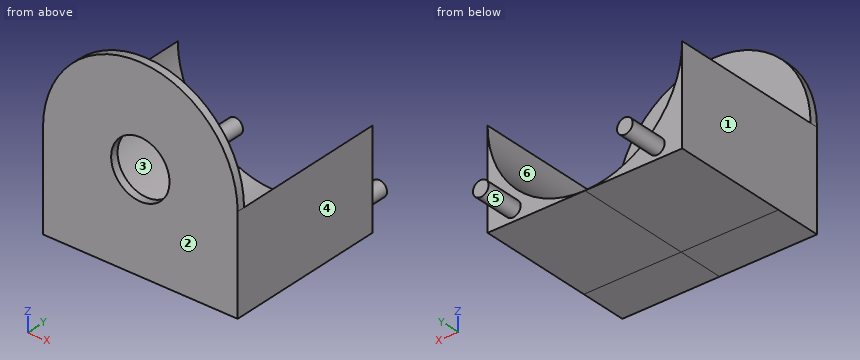
Autodesk Inventor part; units mm, degrees
ref_plane "YZ Plane" through (0, 0, 0) normal (1, 0, 0) x (0, 1, 0)
ref_plane "XZ Plane" through (0, 0, 0) normal (0, 1, 0) x (-1, 0, 0)
ref_plane "XY Plane" through (0, 0, 0) normal (0, 0, 1) x (1, 0, 0)
sketch "Sketch1" plane through (0, 0, 0) normal (0, 1, 0) x (-1, 0, 0)
  circle A0 centre (0, 0) radius 7.5
  circle A1 centre (0, 0) radius 25
  dimension "d0" = 15
  dimension "d1" = 50
extrude "Extrusion1" add sketch "Sketch1" along normal blind 2
sketch "Sketch2" plane through (0, 2, 0) normal (0, 1, 0) x (1, 0, 0)
  circle A0 centre (0, 0) radius 25
  line L0 (25, 0) -> (-25, 0)
  line L1 (-25, 0) -> (-25, 25)
  line L2 (-25, 25) -> (25, 25)
  line L3 (25, 25) -> (25, 0)
  point P0 (0, 25)
extrude "Extrusion2" add sketch "Sketch2" along normal blind 10 and the other way blind 2 contours L1 L2 A0 | A0 L2 L3
sketch "Sketch3" plane through (0, 12, 0) normal (0, 1, 0) x (1, 0, 0)
  circle A0 centre (21.5, 18.5) radius 2
  circle A1 centre (-21.5, 18.5) radius 2
  point P0 (0, 0)
  dimension "d8" = 4
  dimension "d9" = 4
extrude "Extrusion3" add sketch "Sketch3" along normal blind 40
sketch "Sketch4" plane through (0, 0, 0) normal (0, -1, 0) x (1, 0, 0)
  line L0 (25, -25) -> (0, -25)
  arc A0 (25, 0) -> (-25, 0) centre (0, 0) ccw
  line L1 (25, -25) -> (-25, -25)
  line L2 (-25, -25) -> (-25, 0)
  line L3 (-25, 0) -> (25, 0)
  line L4 (25, 0) -> (25, -25)
  arc A1 (0, -25) -> (25, 0) centre (0, 0) ccw
  arc A2 (-25, 0) -> (25, 0) centre (0, 0) ccw
extrude "Extrusion4" add sketch "Sketch4" against normal blind 42 contours L0 A1 L4 | L1 L2 A2
sketch "Sketch5" plane through (21.5, 52, -18.5) normal (0, 1, 0) x (1, 0, 0)
  circle A0 centre (0, 0) radius 2
  circle A1 centre (0, 0) radius 2
  circle A2 centre (-43, 0) radius 2
  circle A3 centre (-43, 0) radius 2
  point P0 (-21.5, -18.5)
extrude "Extrusion5" cut sketch "Sketch5" against normal blind 10
sketch "Sketch6" plane through (0, 42, 0) normal (0, 1, 0) x (1, 0, 0)
  circle A0 centre (18.5, 22) radius 2
  circle A1 centre (-18.5, 22) radius 2
  point P0 (0, 0)
  dimension "d16" = 4
  dimension "d17" = 4
extrude "Extrusion6" add sketch "Sketch6" along normal blind 10
properties part number "trail 3.1" material "Iron, Gray"
Geometry: final body of the model. Coordinates: model frame, mm. Face numbers are marked on the shaded views. A direction names the side the tool comes from. Give positions to 0.01 mm unless a question says otherwise; leave off trailing zeros. Write each loop counter-clockwise with the first axis right and the second up, starting at its lowest first coordinate (ties: lowest second). Pieces come first, ordered by that corner, then holes. Notation, with made-up numbers: (-2, -20.5) -> (11, -20.5) arc R28 cw to (11, -2.5) -> close; hole circle Ø11 at (61.5, 55.25). An arc over 180 degrees is marked (long way). Answer in a Markdown table with one row per item.
(1) Section query C-C on x = -18.5. Return loops of the section in (y, z), then the cut area to 3 significant figures.
Answers below:
| item | result |
|---|---|
| outline | (0, -25) -> (42, -25) -> (42, -24) -> (52, -24) -> (52, -20) -> (42, -20) -> (42, -16.82) -> (2, -16.82) -> (2, 16.82) -> (0, 16.82) -> close |
| area | 451 mm^2 |
(2) Section query D-D on z = -14. Return loops of the section in (x, y), then the cut area to 3 significant figures.
Answers below:
| item | result |
|---|---|
| outline | (-25, 0) -> (25, 0) -> (25, 42) -> (20.71, 42) -> (20.71, 2) -> (-20.71, 2) -> (-20.71, 42) -> (-25, 42) -> close |
| area | 443 mm^2 |
(3) Ray query, line 1 along Z through (x, y) = (0, 1.45); line 2 along Y through (x, z) = (15, 14.5); line 3 along X through (y, z) = (22, -21.5). Return the intervals inside material, ascending. Write a range as [from, to].
Answers below:
| item | result |
|---|---|
| line 1 | [-25, -7.5], [7.5, 25] |
| line 2 | [0, 2] |
| line 3 | [-25, -12.76], [12.76, 25] |
(4) Section query A-A on z = 3. Return loops of the section in (x, y), then the cut area to 3 significant figures.
Answers below:
| item | result |
|---|---|
| outline | (-24.82, 0) -> (-6.87, 0) -> (-6.87, 2) -> (-24.82, 2) -> close; (6.87, 0) -> (24.82, 0) -> (24.82, 2) -> (6.87, 2) -> close |
| area | 71.8 mm^2 |
(5) Pin query (flat end, axial travel): pin 1 (5 mm diameter, centred on x = -11, z = -11.5, fed in from +Y); pin 2 (10 mm diameter, centred on x = 1, y = 25.5, fed in from +Z); pin 3 (12.5 mm diameter, centred on x = -18, z = -11, fed in from +Y). Return the tip coordinate at first contact, or that it passes through.
Answers below:
| item | result |
|---|---|
| pin 1 | y = 2 |
| pin 2 | z = -24.27 |
| pin 3 | y = 42 |
(6) Set-up query: the marked faces 4, 5 and 6. Return all of +Z, -Z, +X, -X, +Y, -Y with unobstructed straight access to the full face (end or side cutting, diameter ignored); none if empty.
Answers below:
| item | result |
|---|---|
| face 4 | +Z, -Z, +X, +Y, -Y |
| face 5 | +Y |
| face 6 | +Z, +Y |
(7) Draft query along X for the marked faces 1, 2 and 3. Return one class per face: +X half, -X half, draft (parallel to the pull), parting line (faces both ways), or undercut.
Answers below:
| item | result |
|---|---|
| face 1 | -X half |
| face 2 | draft |
| face 3 | undercut |
